Build history of the part. All positions in model axes, mm. Coordinates: 2 decimals unless noted, no trailing zeros. Loops run counter-clockwise (first coordinate to the right, second up) from the corner with the lowest first, then second, coordinate; pieces in that order, holes last.
(1) Wall check: L1, parallel to X at y = 5, z = 3.75; L2, parallel to X at y = 5.75, z = 5.75; L3, parallel to Y at x = -6.75, z = 5.25. Give the ranges that are in metal, low to high.
(2) Slice it at C-C (y = 4). Give the cut face in (x, z).
(3) Slice it at A-A (z = 1). Give the cut face in (x, y).
(4) Slice it at B-B (x = -8). Give the cut face in (y, z), and give its area (3 significant figures).
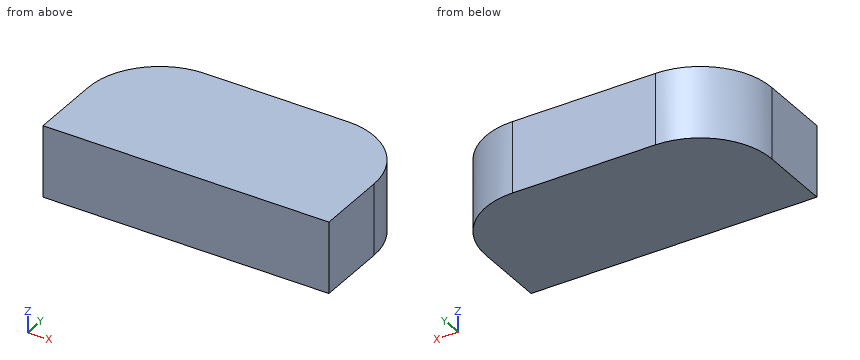
from build123d import *

# Parameters (mm, degrees)
ESQUISSE2_W        = 25.4
ESQUISSE2_H        = 12.7
BOSS_EXTRU_1_DEPTH = 6.35
CONG_1_R           = 6.35


with BuildPart() as part:
    # Esquisse2 → Boss.-Extru.1 (new body)
    with BuildSketch(Plane.XY):
        Rectangle(ESQUISSE2_W, ESQUISSE2_H)
    extrude(amount=BOSS_EXTRU_1_DEPTH)

    # Congé1
    cong_1_edges = [part.edges().sort_by_distance(p)[0] for p in [
        (-12.7, 6.35, 3.175),
        (12.7, 6.35, 3.175),
    ]]
    fillet(cong_1_edges, radius=CONG_1_R)


solid = part.part
Response values:
1. L1: x = -10.26 to 10.26
1. L2: x = -9.04 to 9.04
1. L3: y = -6.35 to 6.34
2. outline: (-11.28, 0) - (11.28, 0) - (11.28, 6.35) - (-11.28, 6.35) - close
3. outline: (-12.7, -6.35) - (12.7, -6.35) - (12.7, 0) arc R6.35 ccw to (6.35, 6.35) - (-6.35, 6.35) arc R6.35 ccw to (-12.7, 0) - close
4. outline: (-6.35, 0) - (6.13, 0) - (6.13, 6.35) - (-6.35, 6.35) - close
4. area: 79.3 mm2
